The listing builds one solid part. Answer for the finished solid, in the listing's coordinates (mm). A direction names the side the tool comes from. Coordinates: 2 decimals unless noted, no trailing zeros. Loops run counter-clockwise (first coordinate to the right, second up) from the corner with the lowest first, then second, coordinate; pieces in that order, holes last. Notation, with made-up numbers: M 62,64.5 L 112,64.5 A12 cw 112,79.5 Z; hole C 32.5,57.25 d3. An arc over 180 degrees is marked long. Answer as a JSON object with one key per item and string values. Group by question number.
1. A cutting plane is placed at A-A on x = 28. Give the vertices of the cut face in (y, z).
2. Determine the mould class of faces 3 (the face through (27.801, -1.847, 0.751)), 4 (the face through (29.182, 0.453, 0.751)), 5 (the face through (23.299, 3.222, 0.751)) for opening direction Y: released by +Y, released by -Y, zero draft, split by the parting line, or undercut.
3. For faces 1 (the face through (23.39, -1.29, 0.75)), 2 (the face through (22, 1.524, 1)), determine the directions among +Z, -Z, +X, -X, +Y, -Y from which every point of the face is accessible in a straight line to the end or side of a thin tool.
4. A cutting plane is placed at B-B on x = 29.75. Give the vertices of the cut face in (y, z).
5. A cutting plane is placed at D-D on y = 0.7. Give the vertices of the cut face in (x, z).
6. Given pin 1 (0.8 mm diameter, centred on y = 0.5, z = 1, fed in from -X), flat-ended and moving along its own axis, determine where the tip first touches the part or whether it passes through.
7. Straight lines are drawn through the part: L1, parallel to Y at x = 22.25, z = 0.9; L2, parallel to Y at x = 21.5, z = 1.25; L3, parallel to Y at x = 25.25, z = 0.85. For each, find the intervals that lie inside material, in ascending order.
8. A cutting plane is placed at C-C on z = 0.85. Give the vertices of the cut face in (x, y), and give its area (3 significant figures).
from build123d import *

# Parameters (mm, degrees)
BOSS_EXTRUDE1_DEPTH = 1.524


with BuildPart() as part:
    # Sketch1 → Boss-Extrude1 (new body)
    with BuildSketch(Plane.XY):
        with BuildLine():
            Line((23.699745488, 1.524), (23.699745488, 0))
            Line((23.699745488, 0), (20.767560847, 0))
            ThreePointArc((20.767560847, 0), (23.42913794, -1.301543103), (26.332873234, -1.890039844))
            ThreePointArc((26.332873234, -1.890039844), (27.822037462, -1.85074691), (29.179825721, -2.463580554))
            ThreePointArc((29.179825721, -2.463580554), (28.364487323, -1.477962315), (27.163224831, -1.038430246))
            ThreePointArc((27.163224831, -1.038430246), (28.728924057, -0.875087412), (30.294623282, -1.038430246))
            ThreePointArc((30.294623282, -1.038430246), (28.84920273, -0.154192624), (27.177608147, 0.123094766))
            ThreePointArc((27.177608147, 0.123094766), (29.209666297, 0.459343802), (31.188707793, 1.03006133))
            ThreePointArc((31.188707793, 1.03006133), (29.188863831, 1.247682511), (27.177608147, 1.207865103))
            ThreePointArc((27.177608147, 1.207865103), (28.357122869, 1.517990015), (29.481047207, 1.991515643))
            ThreePointArc((29.481047207, 1.991515643), (28.187668321, 2.044064099), (26.952298477, 2.430653848))
            ThreePointArc((26.952298477, 2.430653848), (27.921180331, 2.673808335), (28.819454547, 3.110797561))
            ThreePointArc((28.819454547, 3.110797561), (27.535947123, 3.059263221), (26.265619678, 3.249828897))
            ThreePointArc((26.265619678, 3.249828897), (23.258369024, 3.209542673), (20.767560847, 1.524))
            Line((20.767560847, 1.524), (23.699745488, 1.524))
        make_face()
    extrude(amount=BOSS_EXTRUDE1_DEPTH)


solid = part.part
From the geometry:
{
 "1": {"outline": "M -1.89,0 L -1.26,0 L -1.26,1.52 L -1.89,1.52 Z; M -0.91,0 L 0.07,0 L 0.07,1.52 L -0.91,1.52 Z; M 0.23,0 L 1.26,0 L 1.26,1.52 L 0.23,1.52 Z; M 1.41,0 L 2.08,0 L 2.08,1.52 L 1.41,1.52 Z; M 2.7,0 L 3.05,0 L 3.05,1.52 L 2.7,1.52 Z"},
 "2": {"face 3": "released by -Y", "face 4": "undercut", "face 5": "released by +Y"},
 "3": {"face 1": "+Z, -Z, -X, -Y", "face 2": "+Z, -Z, -X"},
 "4": {"outline": "M -0.94,0 L -0.61,0 L -0.61,1.52 L -0.94,1.52 Z; M 0.59,0 L 1.21,0 L 1.21,1.52 L 0.59,1.52 Z"},
 "5": {"outline": "M 23.7,0 L 30.15,0 L 30.15,1.52 L 23.7,1.52 Z"},
 "6": {"pin 1": "stops at x = 23.7"},
 "7": {"L1": "y = -0.83 to 0, 1.52 to 2.77", "L2": "y = -0.44 to 0, 1.52 to 2.26", "L3": "y = -1.76 to 3.43"},
 "8": {"outline": "M 20.77,0 A11.66 ccw 26.33,-1.89 A3.34 cw 29.18,-2.46 A2.45 ccw 27.16,-1.04 A7.59 cw 30.29,-1.04 A4.43 ccw 27.18,0.12 A17.65 ccw 31.19,1.03 A15.7 ccw 27.18,1.21 A8.62 ccw 29.48,1.99 A4.94 cw 26.95,2.43 A4.84 ccw 28.82,3.11 A6.81 cw 26.27,3.25 A5.25 ccw 20.77,1.52 L 23.7,1.52 L 23.7,0 Z", "area": "31.0 mm²"}
}
